```python
from build123d import *

# Parameters (mm, degrees)
SKETCH3_W                                           = 45
SKETCH3_H                                           = 45
SKETCH3_R                                           = 3
BOSS_EXTRUDE2_DEPTH                                 = 7.5
SKETCH5_R                                           = 11.5
CUT_EXTRUDE1_DEPTH                                  = 2.1
CHAMFER1_SIZE                                       = 5
CBORE_FOR_M3_HEX_SOCKET_HEAD_CAP_SCREW1_D           = 3.2
CBORE_FOR_M3_HEX_SOCKET_HEAD_CAP_SCREW1_DEPTH       = 7.5
CBORE_FOR_M3_HEX_SOCKET_HEAD_CAP_SCREW1_CBORE_D     = 6.5
CBORE_FOR_M3_HEX_SOCKET_HEAD_CAP_SCREW1_CBORE_DEPTH = 3.5
SKETCH10_W                                          = 45
SKETCH10_H                                          = 7.5
BOSS_EXTRUDE3_DEPTH                                 = 5
M3_TAPPED_HOLE2_AT_2_COUNT                          = 2
M3_TAPPED_HOLE2_AT_2_PITCH                          = 12


with BuildPart() as part:
    # Sketch3 → Boss-Extrude2 (new body)
    with BuildSketch(Plane(origin=(0, 0, 0), x_dir=(1, 0, 0), z_dir=(0, 1, 0))):
        Rectangle(SKETCH3_W, SKETCH3_H)
        with Locations((0, -1.5)):
            Circle(SKETCH3_R, mode=Mode.SUBTRACT)
    extrude(amount=BOSS_EXTRUDE2_DEPTH)

    # Sketch5 → Cut-Extrude1 (cut)
    with BuildSketch(Plane(origin=(0, 7.5, 0), x_dir=(1, 0, 0), z_dir=(0, 1, 0))):
        with Locations((0, -1.5)):
            Circle(SKETCH5_R)
    extrude(amount=-CUT_EXTRUDE1_DEPTH, mode=Mode.SUBTRACT)

    # Chamfer1
    chamfer1_edges = [part.edges().sort_by_distance(p)[0] for p in [
        (-22.5, 3.75, -22.5),
        (22.5, 3.75, -22.5),
    ]]
    chamfer(chamfer1_edges, length=CHAMFER1_SIZE)

    # CBORE for M3 Hex Socket Head Cap Screw1
    with Locations(Plane(origin=(0, 0, 0), x_dir=(-1, 0, 0), z_dir=(0, -1, 0))):
        with Locations((15.5, 14), (-15.5, -17), (-15.5, 14), (15.5, -17)):
            CounterBoreHole(CBORE_FOR_M3_HEX_SOCKET_HEAD_CAP_SCREW1_D / 2, CBORE_FOR_M3_HEX_SOCKET_HEAD_CAP_SCREW1_CBORE_D / 2, CBORE_FOR_M3_HEX_SOCKET_HEAD_CAP_SCREW1_CBORE_DEPTH, depth=CBORE_FOR_M3_HEX_SOCKET_HEAD_CAP_SCREW1_DEPTH)

    # Sketch10 → Boss-Extrude3 (add)
    with BuildSketch(Plane.XY.offset(22.5)):
        with Locations((0, 3.75)):
            Rectangle(SKETCH10_W, SKETCH10_H)
    extrude(amount=BOSS_EXTRUDE3_DEPTH)

    # Sketch14 → M3 Tapped Hole2 (revolve, cut)
    with BuildSketch(Plane(origin=(-22.5, 3.75, 24), x_dir=(0, 0, 1), z_dir=(0, 1, 0))):
        Polygon((0, 0), (0, 10.751075774), (1.25, 10), (1.25, 0), align=None)
    m3_tapped_hole2 = revolve(axis=Axis((-28.85, 3.75, 24), (1, 0, 0)), mode=Mode.SUBTRACT)

    # M3 Tapped Hole2 at 2: M3 Tapped Hole2 ×2
    with Locations(*[(0, 0, -i * M3_TAPPED_HOLE2_AT_2_PITCH) for i in range(1, M3_TAPPED_HOLE2_AT_2_COUNT)]):
        add(m3_tapped_hole2, mode=Mode.SUBTRACT)

    # Mirror1: M3 Tapped Hole2 across plane
    add(m3_tapped_hole2.mirror(Plane(origin=(0, 0, 0), x_dir=(0, 0, 1), z_dir=(1, 0, 0))), mode=Mode.SUBTRACT)

    # Mirror1 copy 1 sketch → Mirror1 copy 1 (revolve, cut)
    with BuildSketch(Plane(origin=(22.5, 3.75, 12), x_dir=(0, 0, 1), z_dir=(0, 1, 0))):
        Polygon((0, 0), (0, -10.751075774), (1.25, -10), (1.25, 0), align=None)
    revolve(axis=Axis((28.85, 3.75, 12), (1, 0, 0)), mode=Mode.SUBTRACT)


solid = part.part
```
Design review of the part built by this model. Coordinates are the model's own, in mm. A direction names the side the tool comes from. Give positions to 0.01 mm unless a question says otherwise; leave off trailing zeros. Write each loop counter-clockwise with the first axis right and the second up, starting at its lowest first coordinate (ties: lowest second). Pieces come first, ordered by that corner, then holes. Notation, with made-up numbers: (87, 80.5) - (121, 80.5) arc R7 ccw to (121, 87.5) - close; hole circle Ø10 at (30.25, 22). An arc over 180 degrees is marked (long way). Return JSON: item names as keys, results as strings. Group by question number.
(1) Machinability: for faces 1 (the cylindrical face through (17.57, 4.229, 25.155)), 2 (the cylindrical face through (-3, 2.7, 1.4)), 3 (the cylindrical face through (-12.253, 1.726, -14.143)), 4 (the cylindrical face through (-17.57, 4.229, 25.155)), 5 (the flat face through (20, 4, -20)), which of the approach directions +Z, -Z, +X, -X, +Y, -Y give a long, thin tool a straight path to every point of the face, cutting with its end or side? Answer none if there is none.
(2) We need section D-D, the plane z = -14. Give the boundary of the cut face in (x, y), then the cut area to 3 significant figures.
(3) We need section C-C, the plane y = 6. Give the boundary of the cut face in (x, z), then the cut area to 3 significant figures.
(4) We need section A-A, the plane x = 15.5. Give the boundary of the cut face in (y, z), then the cut area to 3 significant figures.
(5) Mouldability with a two-part tool opening along Y and no side actions: class faces 6 (the flat face through (-20, 4, -20)), 7 (the flat face through (-14, 3.5, 18)), 8 (the conical face through (11.88, 3.83, 12.2)) as +Y half, -Y half, draft (parallel to the pull), parting line (faces both ways), or undercut.
(6) To check wall thickness, follow probe 1 along Z at (x, y) = (-15.5, 1.65); probe 2 along Z at (x, y) = (-15.5, 6.45); probe 3 along X at (y, z) = (6.5, 17). State the ranges of each line that lie inside material, in increasing order.
(7) We need section B-B, the plane z = 1.5. Give the boundary of the cut face in (x, y), then the cut area to 3 significant figures.
(8) Insertion check: pin 1 (1 mm diameter, centred on x = -7, z = -3, fed in from +Y); pin 2 (2 mm diameter, centred on y = 3.75, z = 24, fed in from -X); pin 3 (5 mm diameter, centred on x = 15.5, z = 17, fed in from -Y). Each pin has a flat end and moves straight along its axis. Give the tip position at first contact, or say it passes through.
Reported:
{
 "1": {"face 1": "+X", "face 2": "+Y, -Y", "face 3": "-Y", "face 4": "-X", "face 5": "-Z, +X, +Y, -Y"},
 "2": {"outline": "(-22.5, 0) - (-18.75, 0) - (-18.75, 3.5) - (-17.1, 3.5) - (-17.1, 7.5) - (-22.5, 7.5) - close; (-13.9, 3.5) - (-12.25, 3.5) - (-12.25, 0) - (12.25, 0) - (12.25, 3.5) - (13.9, 3.5) - (13.9, 7.5) - (-13.9, 7.5) - close; (17.1, 3.5) - (18.75, 3.5) - (18.75, 0) - (22.5, 0) - (22.5, 7.5) - (17.1, 7.5) - close", "area": "266 mm2"},
 "3": {"outline": "(-22.5, -17.5) - (-17.5, -22.5) - (17.5, -22.5) - (22.5, -17.5) - (22.5, 27.5) - (-22.5, 27.5) - close; hole circle Ø3.2 at (-15.5, -14); hole circle Ø3.2 at (-15.5, 17); hole circle Ø23 at (0, 1.5); hole circle Ø3.2 at (15.5, -14); hole circle Ø3.2 at (15.5, 17)", "area": "1,780 mm2"},
 "4": {"outline": "(0, -22.5) - (7.5, -22.5) - (7.5, -15.6) - (3.5, -15.6) - (3.5, -17.25) - (0, -17.25) - close; (0, -10.75) - (3.5, -10.75) - (3.5, -12.4) - (7.5, -12.4) - (7.5, 15.4) - (3.5, 15.4) - (3.5, 13.75) - (0, 13.75) - close; (0, 20.25) - (3.5, 20.25) - (3.5, 18.6) - (7.5, 18.6) - (7.5, 27.5) - (0, 27.5) - close; hole circle Ø2.5 at (3.75, 12); hole circle Ø2.5 at (3.75, 24)", "area": "294 mm2"},
 "5": {"face 6": "draft", "face 7": "-Y half", "face 8": "undercut"},
 "6": {"probe 1": "z = -22.5 to -17.25, -10.75 to 13.75, 20.25 to 27.5", "probe 2": "z = -22.5 to -15.6, -12.4 to 15.4, 18.6 to 27.5", "probe 3": "x = -22.5 to -17.1, -13.9 to 13.9, 17.1 to 22.5"},
 "7": {"outline": "(-22.5, 0) - (-3, 0) - (-3, 5.4) - (-11.5, 5.4) - (-11.5, 7.5) - (-22.5, 7.5) - close; (3, 0) - (22.5, 0) - (22.5, 7.5) - (11.5, 7.5) - (11.5, 5.4) - (3, 5.4) - close", "area": "257 mm2"},
 "8": {"pin 1": "stops at y = 5.4", "pin 2": "stops at x = -12.35", "pin 3": "stops at y = 3.5"}
}
